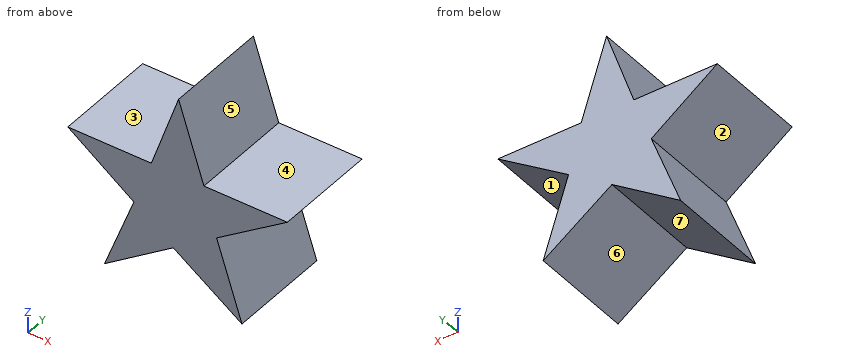
from build123d import *

# Parameters (mm, degrees)
F0_W     = 94.5225581527
F0_H     = 71.0351280868
F1_DEPTH = 25.4
F3_DEPTH = 6.35
F4_DEPTH = 25.4


with BuildPart() as f1:
    # F0 (on Front) → F1 (new body)
    with BuildSketch(Plane.XZ):
        with Locations((6.3969828188, -10.8844134957)):
            Rectangle(F0_W, F0_H)
    extrude(amount=F1_DEPTH)

    # F2 (on face) → F3 (join)
    with BuildSketch(Plane.XZ.offset(25.4)):
        Polygon((0, -3.5492395982), (-25.3826901317, -3.5492395982), (-5.3041339852, -17.9490111768), (-14.2279369757, -41.0697720945), (6.6618728451, -26.8728137016), (27.5516826659, -41.2725880742), (19.8447629809, -17.9490111768), (41.3430146873, -3.5492395982), (15.9913022071, -3.5492395982), (8.2843825221, 19.9771486223), align=None)
    extrude(amount=F3_DEPTH)

    # F4 (cut): a face of the model
    f4_faces = [f1.faces().sort_by_distance(p)[0] for p in [
        (6.3969828188, -25.4, 23.450758759),
    ]]
    extrude(f4_faces, amount=-F4_DEPTH, mode=Mode.SUBTRACT)


solid = f1.part
Can you work these out from the model? Positions are in its coordinate system, mm. Face numbers are marked on the shaded views. A direction names the side the tool comes from. Coordinates: 2 decimals unless noted, no trailing zeros. Loops run counter-clockwise (first coordinate to the right, second up) from the corner with the lowest first, then second, coordinate; pieces in that order, holes last. Notation, with made-up numbers: M -34,-2 L 6,-2 A16 ccw 6,15 Z; hole C -9,44 d2. An arc over 180 degrees is marked long. Answer as CSV lines item,"result". Start each with the question number.
1. If I drill on probe 1 along X at (y, z) = (-5, -33); probe 2 along X at (y, z) = (-28.5, -32); probe 3 along X at (y, z) = (-7.5, -3.5), over which ranges is the centre line in solid material (lowest first)? Write a range as [from, to].
2. For pin 1 Ø5 at (x, y) = (-13, -11) entering from +Z; pin 2 Ø12 at (y, z) = (-8, -21) entering from -X, each with a flat end and sliding along its axis, tell me the tip position at first contact or that it passes through.
3. Suppose I cut it at B-B, the plane z = -36.5. List the corners of the cut face in (x, y) for me, plus the area to 3 significant figures.
4. Suppose I cut it at C-C, the plane y = -8. List the corners of the cut face in (x, z) for me, plus the area to 3 significant figures.
5. For the marked faces 1, 2 and 3, which set-ups out of +Z, -Z, +X, -X, +Y, -Y let a thin tool reach every point of the face, with its end or its side?
6. Thinking about a two-plate mould opening in X: for the marked faces 4, 5, 6 and 7, which applies, +X half, -X half, draft (parallel to the pull), parting line (faces both ways), or undercut?
7. Suppose I cut it at D-D, the plane z = -20. List the corners of the cut face in (x, y) for me, plus the area to 3 significant figures.
8. Suppose I cut it at A-A, the plane x = -12. List the corners of the cut face in (y, z) for me, plus the area to 3 significant figures.
Output:
1,probe 1,"x = [-11.11, -2.35], [15.55, 24.82]"
1,probe 2,"x = [-10.73, -0.88], [14.1, 24.49]"
1,probe 3,"x = [0.02, 15.98]"
2,pin 1,"stops at z = -3.55"
2,pin 2,"stops at x = -9.42"
3,outline,"M -12.46,-31.75 L -7.5,-31.75 L -7.5,0 L -12.46,0 Z; M 20.63,-31.75 L 25.97,-31.75 L 25.97,0 L 20.63,0 Z"
3,area,"327 mm^2"
4,outline,"M -25.38,-3.55 L -5.3,-17.95 L -14.23,-41.07 L 6.66,-26.87 L 27.55,-41.27 L 19.84,-17.95 L 41.34,-3.55 L 15.99,-3.55 L 8.28,19.98 L 0,-3.55 Z"
4,area,"1,330 mm^2"
5,face 1,"+X, +Y, -Y"
5,face 2,"-X, +Y, -Y"
5,face 3,"+Z, -X, +Y, -Y"
6,face 4,"draft"
6,face 5,"+X half"
6,face 6,"undercut"
6,face 7,"undercut"
7,outline,"M -6.1,-31.75 L 20.52,-31.75 L 20.52,0 L -6.1,0 Z"
7,area,"845 mm^2"
8,outline,"M -31.75,-39.56 L 0,-39.56 L 0,-35.3 L -31.75,-35.3 Z; M -31.75,-13.15 L 0,-13.15 L 0,-3.55 L -31.75,-3.55 Z"
8,area,"440 mm^2"
